Check sheet for the drawn part. Datum: minimum x, y, z corner. Units: mm. Give positions to 0.01 mm unless a question says otherwise; leave off trailing zeros. Write each loop counter-clockwise with the first axis right and the second up, starting at its lowest first coordinate (ties: lowest second). Pieces come first, ordered by that corner, then holes. Notation, with made-up numbers: (34.5, 88.25) - (70.5, 88.25) arc R25 ccw to (70.5, 120.25) - close; hole circle Ø1 at (0, -32). An arc over 180 degrees is marked (long way). Answer as a JSON object with one key per item and string values. Group by question number.
Item 1: Sectioned sample at A-A, the plane x = 108. Record the boundary of the cut face in (y, z) (1 decimal).
Item 2: Sectioned sample at B-B, the plane y = 1.1. Count the separate pieces of the cut face and the enclosed holes in it, and give its area (3 significant figures).
Item 3: Sectioned sample at C-C, the plane x = 40.5. Record the boundary of the cut face in (y, z) (1 decimal).
Item 4: Scan lines: line 1 along Z through (x, y) = (86, 2.4) (1 decimal); line 2 along Z through (x, y) = (94, 1.85) (1 decimal); line 3 along X through (y, z) = (1.55, 17) (1 decimal). Record each from-to range of solid material in increasing order. Write a range as [from, to].
Item 5: Go/stop test with flat-tipped pins: pin 1 (1 mm diameter, centred on y = 1.5, z = 36.5, fed in from +X); pin 2 (1 mm diameter, centred on y = 1, z = 35.5, fed in from -X). Record where each tip stops, or that it passes through.
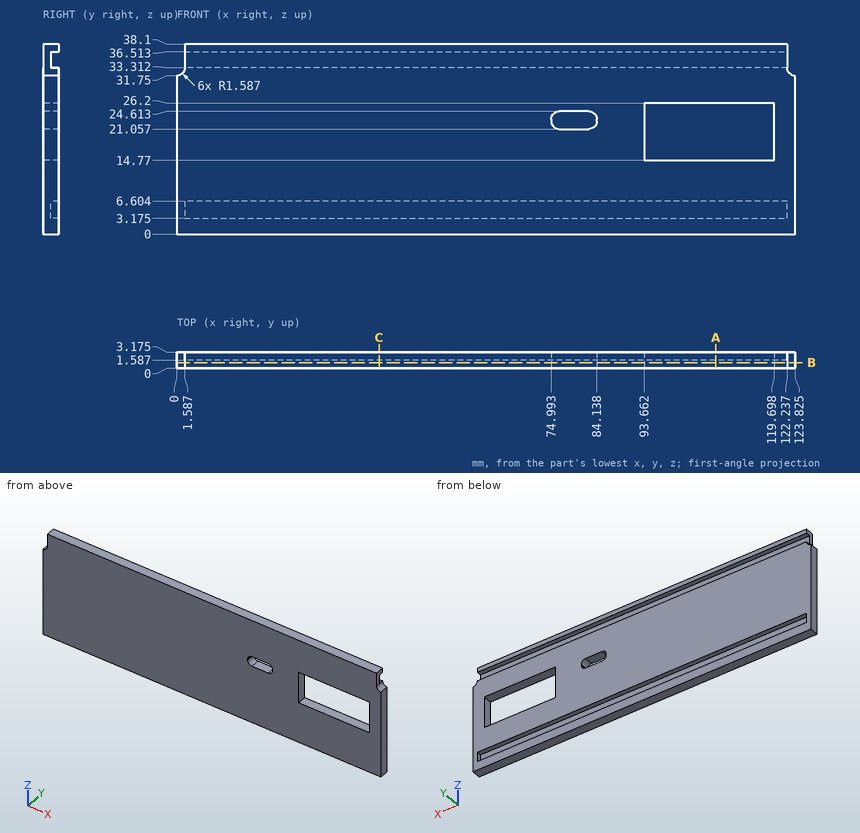
Geometry check:
{
 "1": {"outline": "(0, 0) - (3.2, 0) - (3.2, 3.2) - (1.6, 3.2) - (1.6, 6.6) - (3.2, 6.6) - (3.2, 14.8) - (0, 14.8) - close; (0, 26.2) - (3.2, 26.2) - (3.2, 33.3) - (1.6, 33.3) - (1.6, 36.5) - (3.2, 36.5) - (3.2, 38.1) - (0, 38.1) - close"},
 "2": {"separate pieces": "1", "enclosed holes": "2", "area": "4,370 mm^2"},
 "3": {"outline": "(0, 0) - (3.2, 0) - (3.2, 3.2) - (1.6, 3.2) - (1.6, 6.6) - (3.2, 6.6) - (3.2, 33.3) - (1.6, 33.3) - (1.6, 36.5) - (3.2, 36.5) - (3.2, 38.1) - (0, 38.1) - close"},
 "4": {"line 1": "[0, 3.2], [6.6, 33.3], [36.5, 38.1]", "line 2": "[0, 3.2], [6.6, 14.8], [26.2, 33.3], [36.5, 38.1]", "line 3": "[0, 93.7], [119.7, 123.8]"},
 "5": {"pin 1": "x = 122.24", "pin 2": "x = 1.59"}
}
